For this review, use the dimensioned drawing (mm, ordinates from the lowest corner) and the shaded views. A direction names the side the tool comes from. Round coordinates to 2 decimals unless told otherwise and drop trailing zeros. Order: outer loops, then holes, each group sorted by start corner. A loop starts at its lowest first (then second) coordinate and runs counter-clockwise, first axis right, second up. Notation, with made-up numbers: (-24, -12) -> (13, -12) arc R36 ccw to (13, 26) -> close; hole circle Ø10 at (-12, 79.5). An arc over 180 degrees is marked (long way). Answer in a Markdown table with one row per item.
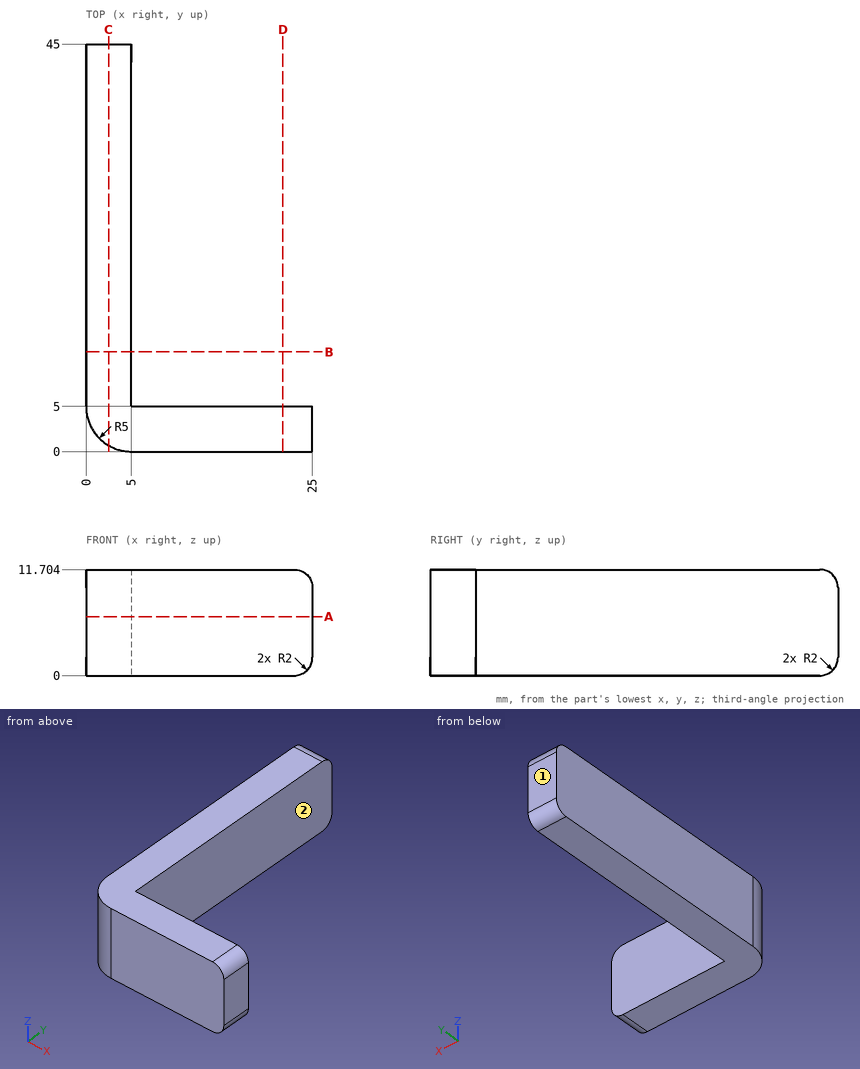
Q1. Clearance check with a flat-ended pin moving along its axis: pin 1 Ø3 at (y, z) = (21.5, 5.5) entering from +X. State where the tip first meets the part, or that it passes through.
Answer key:
| item | result |
|---|---|
| pin 1 | stops at x = 5 |
Q2. Tool access review of the marked faces 1 and 2: name each direction out of +Z, -Z, +X, -X, +Y, -Y from which nothing blocks a thin tool from reaching the whole face with its end or side.
Answer key:
| item | result |
|---|---|
| face 1 | +Z, -Z, +X, -X, +Y |
| face 2 | +Z, -Z, +X, +Y |
Q3. Take a section at B-B, the plane y = 11. Write out the cut boundary in (x, z).
Answer key:
| item | result |
|---|---|
| outline | (0, 0) -> (5, 0) -> (5, 11.7) -> (0, 11.7) -> close |
Q4. Take a section at C-C, the plane x = 2.5. Write out the cut boundary in (y, z).
Answer key:
| item | result |
|---|---|
| outline | (0.67, 0) -> (43, 0) arc R2 ccw to (45, 2) -> (45, 9.7) arc R2 ccw to (43, 11.7) -> (0.67, 11.7) -> close |
Q5. To check wall thickness, follow probe 1 along X at (y, z) = (42.5, 4.25); probe 2 along Y at (x, z) = (1.75, 5.5). State the ranges of each line that lie inside material, in increasing order.
Answer key:
| item | result |
|---|---|
| probe 1 | x = 0 to 5 |
| probe 2 | y = 1.2 to 45 |
Q6. Take a section at A-A, the plane z = 6.5. Write out the cut boundary in (x, y), then the cut area to 3 significant figures.
Answer key:
| item | result |
|---|---|
| outline | (0, 5) arc R5 ccw to (5, 0) -> (25, 0) -> (25, 5) -> (5, 5) -> (5, 45) -> (0, 45) -> close |
| area | 320 mm^2 |
